from build123d import *

# Parameters (mm, degrees)
F1_DEPTH = 25.4


with BuildPart() as f1:
    # F0 (on Front) → F1 (new body)
    with BuildSketch(Plane.XZ):
        with BuildLine():
            Line((203.2, 0), (0, 0))
            Line((0, 0), (21.853262, -31.209693))
            Line((21.853262, -31.209693), (26.014555, -28.295925))
            Line((26.014555, -28.295925), (47.867817, -59.505617))
            Line((47.867817, -59.505617), (43.706524, -62.419386))
            Line((43.706524, -62.419386), (43.706524, -202.119386))
            Line((43.706524, -202.119386), (48.786524, -202.119386))
            Line((48.786524, -202.119386), (48.786524, -341.819386))
            Line((48.786524, -341.819386), (43.706524, -341.819386))
            Line((43.706524, -341.819386), (59.311371, -352.746017))
            Line((59.311371, -352.746017), (62.225139, -348.584725))
            Line((62.225139, -348.584725), (77.829986, -359.511356))
            Line((77.829986, -359.511356), (74.916217, -363.672648))
            ThreePointArc((74.916217, -363.672648), (194.72671, -465.031598), (347.472841, -501.042848))
            Line((347.472841, -501.042848), (336.536605, -490.189096))
            Line((336.536605, -490.189096), (203.2, 0))
        make_face()
    extrude(amount=F1_DEPTH)


solid = f1.part
Check sheet for the modelled part. Datum: model origin and axes. Units: mm. A direction names the side the tool comes from. Give positions to 0.01 mm unless a question says otherwise; leave off trailing zeros. Write each loop counter-clockwise with the first axis right and the second up, starting at its lowest first coordinate (ties: lowest second). Pieces come first, ordered by that corner, then holes. Notation, with made-up numbers: (8.5, 60) -> (33.5, 60) arc R29 cw to (33.5, 84) -> close; hole circle Ø2 at (12.25, 75.5). An arc over 180 degrees is marked (long way). Use one line per item in the form item = value. Start each with the question number.
1. Section check C-C (z = -400.5). Record the cut outline in (x, y).
2. Mould release check, pull along Z, two halves, no side actions. Record for faces 3 (the flat face through (69.918, -12.522, -353.972)), 4 (the cylindrical face through (192.7, -12.5, -464)), 5 (the flat face through (48.787, -13, -271)), 6 (the flat face through (171, 0, -247)): pulls with the +Z half, pulls with the -Z half, needs draft (parallel to the pull), parting line crosses it, or undercut.
3. Section check A-A (y = -7). Record the cut outline in (x, z), and give its area (3 significant figures).
4. Section check B-B (x = 313.5). Record the cut outline in (y, z), and give its area (3 significant figures).
5. Go/stop test with flat-tipped pins: P1, Ø2, axis at y = -14, z = -445.5, coming from the -X side; P2, Ø5, axis at x = 125.5, z = -424.5, coming from the -Y side; P3, Ø3, axis at y = -19.5, z = -272, coming from the +X side; P4, Ø8, axis at y = -14.5, z = -300.5, coming from the +X side. Record where each tip stops, or that it passes through.
6. Thickness scan on line 1 along Z through (x, y) = (77, -9.75); line 2 along Z through (x, y) = (38.5, -4); line 3 along Z through (x, y) = (23.5, -20.5). Record the ranges inside material, lowest first. Write a range as from..to.
7. Access from +Z, -Z, +X, -X, +Y, -Y to the whole of each face (thin tool, end or side, straight path). Record for faces 1 (the flat face through (103, -13, 0)), 2 (the flat face through (43.707, -13, -131)).
Conclusion:
q1.outline = (106.27, -25.4) -> (312.14, -25.4) -> (312.14, 0) -> (106.27, 0) -> close
q2.face_3 = undercut
q2.face_4 = pulls with the -Z half
q2.face_5 = undercut
q2.face_6 = needs draft
q3.outline = (0, 0) -> (21.85, -31.21) -> (26.01, -28.3) -> (47.87, -59.51) -> (43.71, -62.42) -> (43.71, -202.12) -> (48.79, -202.12) -> (48.79, -341.82) -> (43.71, -341.82) -> (59.31, -352.75) -> (62.23, -348.58) -> (77.83, -359.51) -> (74.92, -363.67) arc R336.55 ccw to (347.47, -501.04) -> (336.54, -490.19) -> (203.2, 0) -> close
q3.area = 98,600 mm²
q4.outline = (-25.4, -499.45) -> (0, -499.45) -> (0, -405.5) -> (-25.4, -405.5) -> close
q4.area = 2,390 mm²
q5.P1 = 159.48
q5.P2 = through
q5.P3 = 277.59
q5.P4 = 286.03
q6.line_1 = -366.48..-360.7, -358.93..0
q6.line_2 = -46.13..0
q6.line_3 = -30.06..0
q7.face_1 = +Z, +X, -X, +Y, -Y
q7.face_2 = -Z, -X, +Y, -Y
